Part model, mm, in its own coordinate system. Face numbers are marked on the shaded views. A direction names the side the tool comes from. Give positions to 0.01 mm unless a question says otherwise; leave off trailing zeros. Order: outer loops, then holes, each group sorted by start corner. A loop starts at its lowest first (then second) coordinate and runs counter-clockwise, first axis right, second up. Notation, with made-up numbers: M 44.5,84 L 93.5,84 A19 ccw 93.5,108 Z; hole C 88,5.5 d11. An arc over 180 degrees is marked long. Write each question's results on one line, items separated by ' | '. Start each with the question number.
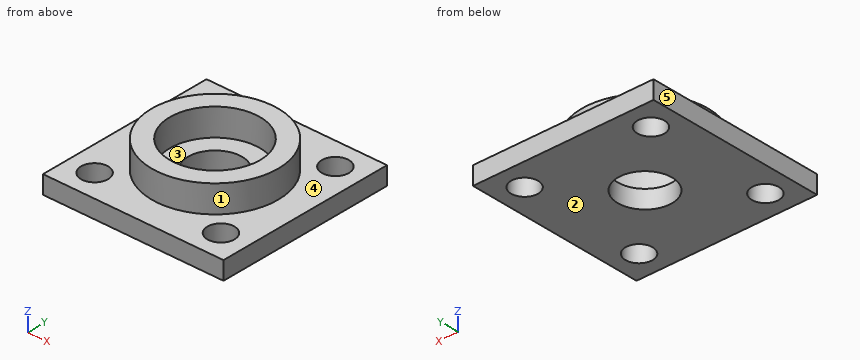
from build123d import *

# Parameters (mm, degrees)
SKETCH_1_W      = 20
SKETCH_1_H      = 20
SKETCH_1_R      = 1.5
SKETCH_1_R_2    = 3
EXTRUDE_1_DEPTH = 2
SKETCH_2_R      = 7
SKETCH_2_R_2    = 5
EXTRUDE_2_DEPTH = 3


with BuildPart() as part:
    # 草图1 → 凸台-拉伸1 (new body)
    with BuildSketch(Plane.XY):
        Rectangle(SKETCH_1_W, SKETCH_1_H)
        with Locations((-7, 7)):
            Circle(SKETCH_1_R, mode=Mode.SUBTRACT)
        with Locations((7, 7)):
            Circle(SKETCH_1_R, mode=Mode.SUBTRACT)
        with Locations((7, -7)):
            Circle(SKETCH_1_R, mode=Mode.SUBTRACT)
        with Locations((-7, -7)):
            Circle(SKETCH_1_R, mode=Mode.SUBTRACT)
        Circle(SKETCH_1_R_2, mode=Mode.SUBTRACT)
    extrude(amount=EXTRUDE_1_DEPTH)

    # 草图2 → 凸台-拉伸2 (add)
    with BuildSketch(Plane.XY.offset(2)):
        Circle(SKETCH_2_R)
        Circle(SKETCH_2_R_2, mode=Mode.SUBTRACT)
    extrude(amount=EXTRUDE_2_DEPTH)


solid = part.part
(1) Saw through at C-C on y = 1.5. Give the cut face in (x, z), plus the area to 3 significant figures.
(2) Tool access for the marked faces 4 and 5: list every direction of +Z, -Z, +X, -X, +Y, -Y with a clear straight run to the whole face (end or side of a thin tool).
(3) Probe L1, parallel to Y at x = 7, z = 1.2; L2, parallel to Y at x = 0, z = 3.05; L3, parallel to Y at x = 0, z = 0.9. List the from-to ranges inside material, lowest first.
(4) Saw through at B-B on z = 1.6. Give the cut face in (x, y).
(5) Drop flat-ended pins along their axis: P1, Ø4, axis at x = 7, y = -7, coming from the +Z side; P2, Ø3, axis at x = -7, z = 4, coming from the -Y side. Give the stop position or say it passes through.
(6) Pull direction Y, two halves, no side cores. Call the marked faces 1, 2 and 3: +Y half, -Y half, draft (parallel to the pull), parting line (faces both ways), or undercut.
(7) Saw through at D-D on z = 3.9. Give the cut face in (x, y).
(8) Saw through at A-A on x = 0. Give the cut face in (y, z), plus the area to 3 significant figures.
Taken from the geometry:
1) outline: M -10,0 L -2.6,0 L -2.6,2 L -4.77,2 L -4.77,5 L -6.84,5 L -6.84,2 L -10,2 Z; M 2.6,0 L 10,0 L 10,2 L 6.84,2 L 6.84,5 L 4.77,5 L 4.77,2 L 2.6,2 Z | area: 42.0 mm²
2) face 4: +Z | face 5: +Z, -Z, -X, +Y, -Y
3) L1: y = -10 to -8.5, -5.5 to 5.5, 8.5 to 10 | L2: y = -7 to -5, 5 to 7 | L3: y = -10 to -3, 3 to 10
4) outline: M -10,-10 L 10,-10 L 10,10 L -10,10 Z; hole C -7,-7 d3; hole C -7,7 d3; hole C 0,0 d6; hole C 7,-7 d3; hole C 7,7 d3
5) P1: stops at z = 2 | P2: stops at y = -4.33
6) face 1: parting line | face 2: draft | face 3: undercut
7) outline: C 0,0 d14; hole C 0,0 d10
8) outline: M -10,0 L -3,0 L -3,2 L -5,2 L -5,5 L -7,5 L -7,2 L -10,2 Z; M 3,0 L 10,0 L 10,2 L 7,2 L 7,5 L 5,5 L 5,2 L 3,2 Z | area: 40.0 mm²
